Verification items for the finished model (mm, model axes). A direction names the side the tool comes from. Give positions to 0.01 mm unless a question says otherwise; leave off trailing zeros. Loops run counter-clockwise (first coordinate to the right, second up) from the corner with the lowest first, then second, coordinate; pieces in that order, holes last. Notation, with made-up numbers: M 45,16 L 71,16 A9 cw 71,26 Z; hole C 60,87.25 d5. An arc over 180 degrees is marked long. Use a Markdown table: item, result.
from build123d import *

# Parameters (mm, degrees)
SKETCH1_R           = 254
SKETCH1_R_2         = 233.38
BOSS_EXTRUDE1_DEPTH = 2250
CUT_EXTRUDE1_REACH  = 256
SKETCH2_R           = 57.25
CUT_EXTRUDE2_REACH  = 256
SKETCH3_R           = 57.25
CUT_EXTRUDE3_REACH  = 256
SKETCH4_R           = 24.5
SKETCH5_W           = 200
SKETCH5_H           = 10
REVOLVE1_ANGLE      = 16
SKETCH6_R           = 30
BOSS_EXTRUDE2_DEPTH = 4


with BuildPart() as part:
    # Sketch1 → Boss-Extrude1 (new body)
    with BuildSketch(Plane.XY):
        Circle(SKETCH1_R)
        Circle(SKETCH1_R_2, mode=Mode.SUBTRACT)
    extrude(amount=-BOSS_EXTRUDE1_DEPTH)

    # Sketch2 → Cut-Extrude1 (cut, up to next)
    with BuildSketch(Plane(origin=(0, 0, 0), x_dir=(1, 0, 0), z_dir=(0, 1, 0)), mode=Mode.PRIVATE) as cut_extrude1_sk1:
        with Locations((0, 179)):
            Circle(SKETCH2_R)
    cut_extrude1_tool1 = extrude(cut_extrude1_sk1.sketch, amount=CUT_EXTRUDE1_REACH, mode=Mode.PRIVATE) & part.part
    add(cut_extrude1_tool1.solids().sort_by_distance((0, 0, -179))[0], mode=Mode.SUBTRACT)

    # Sketch3 → Cut-Extrude2 (cut, up to next)
    with BuildSketch(Plane(origin=(0, 0, 0), x_dir=(1, 0, 0), z_dir=(0, 1, 0)), mode=Mode.PRIVATE) as cut_extrude2_sk1:
        with Locations((0, 2049)):
            Circle(SKETCH3_R)
    cut_extrude2_tool1 = extrude(cut_extrude2_sk1.sketch, amount=-CUT_EXTRUDE2_REACH, mode=Mode.PRIVATE) & part.part
    add(cut_extrude2_tool1.solids().sort_by_distance((0, 0, -2049))[0], mode=Mode.SUBTRACT)

    # Sketch4 → Cut-Extrude3 (cut, up to next)
    with BuildSketch(Plane(origin=(0, 0, 0), x_dir=(1, 0, 0), z_dir=(0, 1, 0)), mode=Mode.PRIVATE) as cut_extrude3_sk1:
        with Locations((0, 649)):
            Circle(SKETCH4_R)
    cut_extrude3_tool1 = extrude(cut_extrude3_sk1.sketch, amount=-CUT_EXTRUDE3_REACH, mode=Mode.PRIVATE) & part.part
    add(cut_extrude3_tool1.solids().sort_by_distance((0, 0, -649))[0], mode=Mode.SUBTRACT)

    # Sketch5 → Revolve1 (revolve, symmetric)
    with BuildSketch(Plane(origin=(0, 0, 0), x_dir=(0, 0, -1), z_dir=(1, 0, 0))) as revolve1_sk:
        with Locations((479, 259)):
            Rectangle(SKETCH5_W, SKETCH5_H)
        with Locations((1879, 259)):
            Rectangle(SKETCH5_W, SKETCH5_H)
    revolve(axis=Axis((0, 0, 0), (0, 0, -1)), revolution_arc=REVOLVE1_ANGLE / 2)
    revolve(revolve1_sk.sketch, axis=Axis((0, 0, 0), (0, 0, 1)), revolution_arc=REVOLVE1_ANGLE / 2)

    # Sketch6 → Boss-Extrude2 (add, symmetric)
    with BuildSketch(Plane(origin=(0, 0, 0), x_dir=(0, 0, -1), z_dir=(1, 0, 0))):
        with BuildLine():
            Line((479, 251.52808946), (569, 251.52808946))
            Line((569, 251.52808946), (569, 306.52808946))
            Line((569, 306.52808946), (530.784861392, 371.832018754))
            ThreePointArc((530.784861392, 371.832018754), (479, 401.52808946), (427.215138608, 371.832018754))
            Line((427.215138608, 371.832018754), (389, 306.52808946))
            Line((389, 306.52808946), (389, 251.52808946))
            Line((389, 251.52808946), (479, 251.52808946))
        make_face()
        with Locations((479, 341.52808946)):
            Circle(SKETCH6_R, mode=Mode.SUBTRACT)
        with BuildLine():
            Line((1969, 251.52808946), (1969, 306.52808946))
            Line((1969, 306.52808946), (1930.784861392, 371.832018754))
            ThreePointArc((1930.784861392, 371.832018754), (1879, 401.52808946), (1827.215138608, 371.832018754))
            Line((1827.215138608, 371.832018754), (1789, 306.52808946))
            Line((1789, 306.52808946), (1789, 251.52808946))
            Line((1789, 251.52808946), (1879, 251.52808946))
            Line((1879, 251.52808946), (1969, 251.52808946))
        make_face()
        with Locations((1879, 341.52808946)):
            Circle(SKETCH6_R, mode=Mode.SUBTRACT)
    extrude(amount=BOSS_EXTRUDE2_DEPTH, both=True)


solid = part.part
(1) Cross-section at A-A on z = -1879. Record the cut outline in (x, y), then the cut area to 3 significant figures.
Results below:
| item | result |
|---|---|
| outline | M -36.74,261.43 L -35.35,251.53 A254 ccw long 35.35,251.53 L 36.74,261.43 A264 ccw 4,263.97 L 4,311.53 L -4,311.53 L -4,263.97 A264 ccw Z; M -4,371.53 L 4,371.53 L 4,401.53 L -4,401.53 Z; hole C 0,0 d466.76 |
| area | 32,900 mm^2 |
(2) Material ranges on line 1 (Y direction, x = 13.5, z = -477.5); line 2 (Y direction, x = 3.5, z = -1568); line 3 (X direction, y = 4.5, z = -1022.5), recorded low to high.
Results below:
| item | result |
|---|---|
| line 1 | -253.64 to -232.99, 232.99 to 263.65 |
| line 2 | -253.98 to -233.35, 233.35 to 253.98 |
| line 3 | -253.96 to -233.34, 233.34 to 253.96 |
(3) Draft check along Y on faces 5 (the cylindrical face through (-0.056, 330.038, -1906.712)), 6 (the flat face through (0.056, 339.637, -1808.375)), 7 (the cylindrical face through (-50.59, -227.83, -1109.25)), 8 (the flat face through (4, 303, -478)). Enter one of: +Y half, -Y half, draft (parallel to the pull), parting line (faces both ways), or undercut.
Results below:
| item | result |
|---|---|
| face 5 | undercut |
| face 6 | +Y half |
| face 7 | undercut |
| face 8 | draft |
(4) Set-up check for faces 1 (the cylindrical face through (-12.41, 239.93, -123.11)), 2 (the flat face through (-4, 303, -1878)), 3 (the cylindrical face through (-12.41, -239.93, -1993.11)), 4 (the flat face through (4, 303, -1878)): record each of +Z, -Z, +X, -X, +Y, -Y from which the full face is reachable in a straight line by a thin tool's end or side.
Results below:
| item | result |
|---|---|
| face 1 | +Y |
| face 2 | +Z, -Z, -X, +Y |
| face 3 | -Y |
| face 4 | +Z, -Z, +X, +Y |
(5) Cross-section at B-B on x = -205.5. Record the cut outline in (y, z), then the cut area to 3 significant figures.
Results below:
| item | result |
|---|---|
| outline | M -149.28,-2250 L -110.62,-2250 L -110.62,0 L -149.28,0 Z; M 110.62,-2250 L 149.28,-2250 L 149.28,0 L 110.62,0 Z |
| area | 174,000 mm^2 |
(6) Cross-section at D-D on z = -825. Record the cut outline in (x, y).
Results below:
| item | result |
|---|---|
| outline | C 0,0 d508; hole C 0,0 d466.76 |
(7) Gauge pin test, flat ends, axial feed: P1, Ø4, axis at x = 145.5, z = -1041.5, coming from the +Y side; P2, Ø2.5, axis at x = -1, y = 289, coming from the -Z side; P3, Ø8, axis at x = -93, z = -273, coming from the +Y side; P4, Ø1.5, axis at x = 153.5, y = 195, coming from the +Z side. Record the tip position at first contact, or that the pin passes through.
Results below:
| item | result |
|---|---|
| P1 | y = 209.58 |
| P2 | z = -1969 |
| P3 | y = 237.9 |
| P4 | z = 0 |
(8) Cross-section at C-C on y = -148.5. Record the cut outline in (x, z), then the cut area to 3 significant figures.
Results below:
| item | result |
|---|---|
| outline | M -206.07,-2250 L -180.04,-2250 L -180.04,0 L -206.07,0 Z; M 180.04,-2250 L 206.07,-2250 L 206.07,0 L 180.04,0 Z |
| area | 117,000 mm^2 |
